Design review of the part shown in the three views and the two pictorial views. Dimensions are in mm from the part's minimum x, y and z. Round coordinates to 2 decimals unless told otherwise and drop trailing zeros.
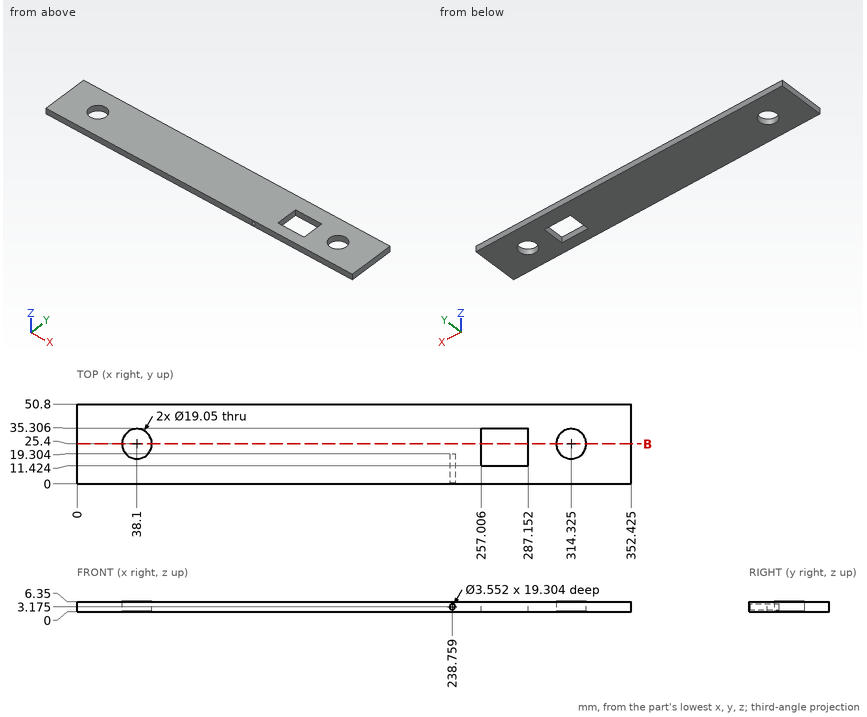
(1) To check wall thickness, follow probe 1 along Y at (x, z) = (38.1, 2.5) (1 decimal); probe 2 along X at (y, z) = (29.5, 5.5) (1 decimal); probe 3 along X at (y, z) = (12, 5.5) (1 decimal). State the ranges of each line that lie inside material, in increasing order.
Data:
probe 1: y = 0 to 15.9, 34.9 to 50.8
probe 2: x = 0 to 29.5, 46.7 to 257, 287.2 to 305.7, 322.9 to 352.4
probe 3: x = 0 to 257, 287.2 to 352.4
(2) Consider section B-B (y = 25.4). State how many separate pieces and enclosed holes the cut face has.
Data:
separate pieces: 4
enclosed holes: 0
(3) Insertion check: pin 1 (11.5 mm diameter, centred on x = 314.325, y = 25.4, fed in from -Z); pin 2 (1.8 mm diameter, centred on x = 238, z = 3.5, fed in from -Y). Each pin has a flat end and moves straight along its axis. Give the tip position at first contact, or say it passes through.
Data:
pin 1: passes through
pin 2: stops at y = 19.3
